Autodesk Fusion 360 part; units mm, degrees
sketch "Sketch1" plane through (0, 0, 0) normal (0, 0, 1) x (1, 0, 0)
  line L0 (-47.5, 47.5) -> (47.5, 47.5)
  line L1 (47.5, 47.5) -> (47.5, -47.5)
  line L2 (47.5, -47.5) -> (-47.5, -47.5)
  line L3 (-47.5, -47.5) -> (-47.5, 47.5)
  line L4 (-47.5, 47.5) -> (47.5, -47.5) construction
  line L5 (-47.5, -47.5) -> (47.5, 47.5) construction
  circle A0 centre (0, 0) radius 35.2
  dimension "d1" = 95
  dimension "d2" = 95
  dimension "d3" = 70.4
extrude "Extrude1" add sketch "Sketch1" along normal blind 10
sketch "Sketch2" plane through (0, 0, 10) normal (0, 0, 1) x (-1, 0, 0)
  circle A0 centre (0, 0) radius 35.2
  line L0 (47.5, 47.5) -> (-47.5, 47.5)
  line L1 (-47.5, 47.5) -> (-47.5, -47.5)
  line L2 (-47.5, -47.5) -> (47.5, -47.5)
  line L3 (47.5, -47.5) -> (47.5, 47.5)
  line L4 (42.5, 0) -> (-42.5, 0) construction
  line L5 (0, -42.5) -> (0, 42.5) construction
  point P0 (0, -42.5)
  point P1 (42.5, 0)
  point P2 (0, 42.5)
  point P3 (-42.5, 0)
  dimension "d7" = 5
  dimension "d8" = 5
  dimension "d9" = 5
  dimension "d10" = 5
hole "Hole1" at (-42.5, 0, 10) at (0, 42.5, 10) at (42.5, 0, 10) at (0, -42.5, 10) direction (0, 0, -1) diameter 4.5 depth 15 tip angle 118 counterbore diameter 8 counterbore depth 4
sketch "Sketch3" plane through (0, 0, 10) normal (0, 0, 1) x (-1, 0, 0)
  circle A0 centre (-42.5, 0) radius 4
  circle A1 centre (42.5, 0) radius 4
  circle A2 centre (0, -42.5) radius 4
  circle A3 centre (0, 42.5) radius 4
  circle A4 centre (0, 0) radius 35.2
  line L0 (47.5, 47.5) -> (-47.5, 47.5)
  line L1 (-47.5, 47.5) -> (-47.5, -47.5)
  line L2 (-47.5, -47.5) -> (47.5, -47.5)
  line L3 (47.5, -47.5) -> (47.5, 47.5)
  circle A5 centre (0, 0) radius 35.2
  circle A6 centre (0, 0) radius 37.2
  dimension "d16" = 2
extrude "Extrude2" add sketch "Sketch3" along normal blind 52 contours A6
sketch "Sketch4" plane through (0, 0, 10) normal (0, 0, 1) x (-1, 0, 0)
  circle A0 centre (0, 0) radius 37.2
  circle A1 centre (-42.5, 0) radius 4
  circle A2 centre (42.5, 0) radius 4
  circle A3 centre (0, -42.5) radius 4
  circle A4 centre (0, 42.5) radius 4
  line L0 (47.5, 47.5) -> (-47.5, 47.5)
  line L1 (-47.5, 47.5) -> (-47.5, -47.5)
  line L2 (-47.5, -47.5) -> (47.5, -47.5)
  line L3 (47.5, -47.5) -> (47.5, 47.5)
  line L4 (37.5, -37.5) -> (-37.5, -37.5) construction
  line L5 (-37.5, -37.5) -> (-37.5, 37.5) construction
  line L6 (-37.5, 37.5) -> (37.5, 37.5) construction
  line L7 (37.5, 37.5) -> (37.5, -37.5) construction
  point P0 (37.5, -37.5)
  point P1 (-37.5, -37.5)
  point P2 (-37.5, 37.5)
  point P3 (37.5, 37.5)
  dimension "d19" = 10
  dimension "d20" = 10
  dimension "d21" = 10
  dimension "d22" = 10
hole "Hole2" at (-37.5, -37.5, 10) at (-37.5, 37.5, 10) at (37.5, 37.5, 10) at (37.5, -37.5, 10) direction (0, 0, -1) diameter 11 end through all
equation "d2 = d1"
equation "d8 = d7"
equation "d9 = d7"
equation "d10 = d7"
equation "d20 = d19"
equation "d21 = d19"
equation "d22 = d19"
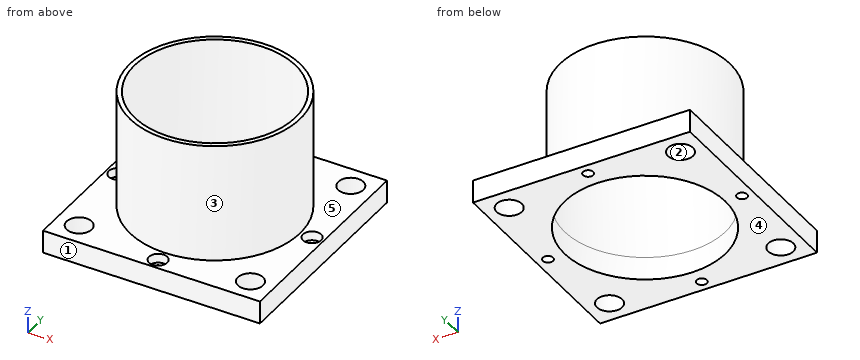
Verification items for the finished model (mm, model axes). Face numbers are marked on the shaded views. A direction names the side the tool comes from. Coordinates: 2 decimals unless noted, no trailing zeros. Order: outer loops, then holes, each group sorted by start corner. A loop starts at its lowest first (then second) coordinate and runs counter-clockwise, first axis right, second up. Notation, with made-up numbers: M 31.5,76 L 35.5,76 A20 ccw 35.5,107 Z; hole C 34,66 d2. An arc over 180 degrees is marked long. Return JSON: item names as keys, results as strings.
1) Cross-section at A-A, the plane x = 0. Record the boundary of the cut face in (y, z), and give its area (3 significant figures).
Answer list:
{"outline": "M -47.5,0 L -44.75,0 L -44.75,6 L -46.5,6 L -46.5,10 L -47.5,10 Z; M -40.25,0 L -35.2,0 L -35.2,62 L -37.2,62 L -37.2,10 L -38.5,10 L -38.5,6 L -40.25,6 Z; M 35.2,0 L 40.25,0 L 40.25,6 L 38.5,6 L 38.5,10 L 37.2,10 L 37.2,62 L 35.2,62 Z; M 44.75,0 L 47.5,0 L 47.5,10 L 46.5,10 L 46.5,6 L 44.75,6 Z", "area": "336 mm2"}
2) Cross-section at B-B, the plane y = -10. Record the boundary of the cut face in (x, z).
Answer list:
{"outline": "M -47.5,0 L -33.75,0 L -33.75,62 L -35.83,62 L -35.83,10 L -47.5,10 Z; M 33.75,0 L 47.5,0 L 47.5,10 L 35.83,10 L 35.83,62 L 33.75,62 Z"}
3) Release check for a two-part mould opening along X. For the marked faces 1, 2 and 3 record: +X half, -X half, draft (parallel to the pull), parting line (faces both ways), or undercut.
Answer list:
{"face 1": "draft", "face 2": "undercut", "face 3": "parting line"}
4) Thickness scan on L1, parallel to Y at x = -37, z = 7; L2, parallel to X at y = 0, z = 9.1. Record the ranges inside material, lowest first. Write a range as [from, to].
Answer list:
{"L1": "[-47.5, -42.98], [-32.02, 32.02], [42.98, 47.5]", "L2": "[-47.5, -46.5], [-38.5, -35.2], [35.2, 38.5], [46.5, 47.5]"}
5) Cross-section at C-C, the plane z = 14. Record the boundary of the cut face in (x, y).
Answer list:
{"outline": "C 0,0 d74.4; hole C 0,0 d70.4"}
6) Gauge pin test, flat ends, axial feed: pin 1 (9 mm diameter, centred on x = 37.5, y = -37.5, fed in from +Z); pin 2 (4 mm diameter, centred on x = -41, y = 1, fed in from +Z); pin 3 (17.5 mm diameter, centred on x = -37.5, y = -37.5, fed in from -Z); pin 4 (4 mm diameter, centred on x = -24.5, y = 36, fed in from +Z). Record the tip position at first contact, or that the pin passes through.
Answer list:
{"pin 1": "through", "pin 2": "z = 6", "pin 3": "z = 0", "pin 4": "z = 10"}
7) Cross-section at D-D, the plane y = -20. Record the boundary of the cut face in (x, z).
Answer list:
{"outline": "M -47.5,0 L -28.97,0 L -28.97,62 L -31.37,62 L -31.37,10 L -47.5,10 Z; M 28.97,0 L 47.5,0 L 47.5,10 L 31.37,10 L 31.37,62 L 28.97,62 Z"}
8) Access from +Z, -Z, +X, -X, +Y, -Y to the whole of each face (thin tool, end or side, straight path). Record for the marked faces 4 and 5.
Answer list:
{"face 4": "-Z, +X, -X, +Y, -Y", "face 5": "+Z"}
